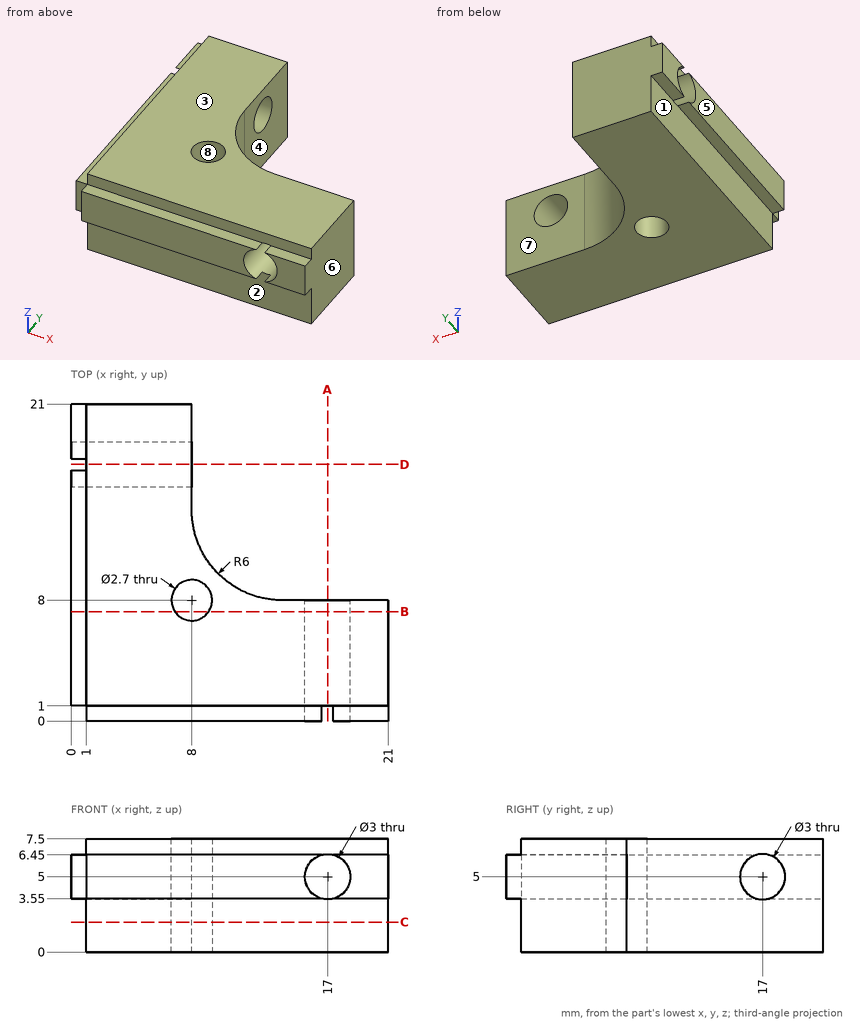
For this review, use the dimensioned drawing (mm, ordinates from the lowest corner) and the shaded views. A direction names the side the tool comes from. Give positions to 0.01 mm unless a question says otherwise; leave off trailing zeros. Loops run counter-clockwise (first coordinate to the right, second up) from the corner with the lowest first, then second, coordinate; pieces in that order, holes last. Notation, with made-up numbers: (1, 25.25) -> (28, 25.25) arc R20 cw to (28, 44.25) -> close; hole circle Ø7 at (63.25, 13). An arc over 180 degrees is marked (long way). One line per question, with ' | ' between items. Start each with the question number.
(1) Insertion check: P1, Ø1.1, axis at x = 20, y = 0.5, coming from the -Z side; P2, Ø0.8, axis at x = 0.5, y = 19, coming from the -Z side; P3, Ø3.5, axis at y = 16.5, z = 3, coming from the +X side; P4, Ø0.5, axis at x = 0.5, y = 20, coming from the +Z side. Each pin has a flat end and moves straight along its axis. Give the tip position at first contact, or say it passes through.
(2) We need section A-A (x = 17). State the section outline as (y, z) points.
(3) For the marked faces 1, 2, 3, 4 and 5, list the 3-axis set-ups (+Z, -Z, +X, -X, +Y, -Y) from which the entire face can be reached by the end or side of a thin tool; tool diameter is ignored.
(4) Draft analysis for pull direction X (two halves, no side actions). For the marked faces 6, 7 and 8, state which applies: +X half, -X half, draft (parallel to the pull), parting line (faces both ways), or undercut.
(5) We need section C-C (z = 2). State the section outline as (x, y) points, and give its area (3 significant figures).
(6) For line 1 (Z direction, x = 17, y = 3.5); line 2 (Y direction, x = 7.75, z = 5.5); line 3 (X direction, y = 4.5, z = 1.75), list the stretches that pass through material, from the lowest coordinate up.
(7) We need section B-B (y = 7.25). State the section outline as (x, z) points, and give its area (3 significant figures).
The answers:
1) P1: stops at z = 0 | P2: stops at z = 3.55 | P3: stops at x = 8 | P4: stops at z = 6.45
2) outline: (1, 0) -> (8, 0) -> (8, 3.5) -> (1, 3.5) -> close; (1, 6.5) -> (8, 6.5) -> (8, 7.5) -> (1, 7.5) -> close
3) face 1: -Z, -X, +Y, -Y | face 2: -Z, +X, -X, -Y | face 3: +Z, +X, -X, +Y, -Y | face 4: +Z, -Z, +X, +Y | face 5: +Z, -Z, -X, +Y, -Y
4) face 6: +X half | face 7: draft | face 8: undercut
5) outline: (1, 1) -> (21, 1) -> (21, 8) -> (14, 8) arc R6 cw to (8, 14) -> (8, 21) -> (1, 21) -> close; hole circle Ø2.7 at (8, 8) | area: 233 mm^2
6) line 1: z = 0 to 3.5, 6.5 to 7.5 | line 2: y = 0 to 6.67, 9.33 to 15.59, 18.41 to 21 | line 3: x = 1 to 21
7) outline: (0, 3.55) -> (1, 3.55) -> (1, 0) -> (6.88, 0) -> (6.88, 7.5) -> (1, 7.5) -> (1, 6.45) -> (0, 6.45) -> close; (9.12, 0) -> (21, 0) -> (21, 7.5) -> (9.12, 7.5) -> close; hole circle Ø3 at (17, 5) | area: 129 mm^2
